Could you check a few things on this model? Use its own coordinates, in mm. A direction names the side the tool comes from. Round coordinates to 2 decimals unless told otherwise and drop trailing zeros. Loops run counter-clockwise (first coordinate to the right, second up) from the corner with the lowest first, then second, coordinate; pieces in that order, holes last. Notation, with made-up numbers: (-18, 38.5) -> (26, 38.5) arc R16 ccw to (26, 50.5) -> close; hole circle Ø5 at (26, 49.25). An arc over 180 degrees is marked (long way). Write each question's results on one line, items separated by ' | '. Start each with the question number.
1) Imagine slicing it at A-A, the plane y = 4.5. List the corners of the cut face in (x, z) for me.
2) Which directions (+Z, -Z, +X, -X, +Y, -Y) give clear straight access to the entire face, cutting with the end or side of a thin tool? Please do faces 4 (the flat face through (-2.642, 1, -7)), 5 (the flat face through (8, 9, -1.016)), 6 (the flat face through (6.706, 9.1, -0.5)).
3) Imagine slicing it at D-D, the plane z = -6. List the corners of the cut face in (x, y) for me.
4) For P1, Ø2, axis at x = 2, z = -3, coming from the +Y side, with a flat end and sliding along its axis, tell me the tip position at first contact or that it passes through.
5) If I drill on probe 1 along Z at (x, y) = (8.75, 11.5); probe 2 along Z at (x, y) = (4, 3.25); probe 3 along Y at (x, z) = (-1.5, -4), over which ranges is the centre line in solid material (lowest first)?
6) Imagine slicing it at C-C, the plane z = -0.25. List the corners of the cut face in (x, y) for me (3 decimals).
7) Imagine slicing it at B-B, the plane x = 1.5. List the corners of the cut face in (y, z) for me (3 decimals), plus the area to 3 significant figures.
8) We'd pull the mould along Z, two halves only. Please class faces 1 (the flat face through (-1, 9, -11.684)), 2 (the flat face through (3, 8, 5.08)), 3 (the flat face through (3, 0, -7)): pulls with the +Z half, pulls with the -Z half, needs draft (parallel to the pull), parting line crosses it, or undercut.
Autodesk Inventor part; units mm, degrees
ref_plane "YZ Plane" through (0, 0, 0) normal (1, 0, 0) x (0, 1, 0)
ref_plane "XZ Plane" through (0, 0, 0) normal (0, 1, 0) x (-1, 0, 0)
ref_plane "XY Plane" through (0, 0, 0) normal (0, 0, 1) x (1, 0, 0)
sketch "Sketch5" plane through (0, 0, 0) normal (0, 1, 0) x (-1, 0, 0)
  line L0 (0, 0) -> (-6.604, 0) construction
  line L1 (-6.604, 0) -> (-6.604, -12.7) construction
  line L2 (-6.604, -12.7) -> (0, -12.7) construction
  line L3 (0, -12.7) -> (0, 0) construction
  line L4 (2.6416, -15.24) -> (-9.2456, -15.24)
  line L5 (-9.2456, -15.24) -> (-9.2456, 2.54)
  line L6 (-9.2456, 2.54) -> (2.6416, 2.54)
  line L7 (2.6416, 2.54) -> (2.6416, -15.24)
  dimension "d22" = 6.604
  dimension "d23" = 12.7
  dimension "d24" = 2.6416
  dimension "d25" = 2.6416
  dimension "d26" = 2.54
  dimension "d27" = 2.54
extrude "Extrusion3" add sketch "Sketch5" along normal blind 2.54
sketch "Sketch6" plane through (0, 2.54, 0) normal (0, 1, 0) x (1, 0, 0)
  line L0 (-2.6416, -2.54) -> (9.2456, -2.54)
  line L1 (9.2456, -2.54) -> (9.2456, 0)
  line L2 (6.7056, 0) -> (-0.1016, 0)
  line L3 (-2.6416, -0.508) -> (-2.6416, -2.54)
  line L4 (-2.6416, 15.24) -> (-2.6416, -2.54)
  line L5 (9.2456, -2.54) -> (9.2456, 15.24)
  line L6 (-2.6416, -2.54) -> (9.2456, -2.54)
  line L7 (-0.1016, 12.7) -> (6.7056, 12.7)
  line L8 (9.2456, 12.954) -> (9.2456, 15.24)
  line L9 (9.2456, 15.24) -> (-2.6416, 15.24)
  line L10 (-2.6416, 15.24) -> (-2.6416, 12.7)
  line L11 (9.2456, 15.24) -> (-2.6416, 15.24)
  line L12 (9.2456, 12.954) -> (9.2456, 11.684)
  line L13 (6.7056, 11.684) -> (6.7056, 12.7)
  line L14 (6.7056, 11.684) -> (9.2456, 11.684)
  line L15 (-2.6416, 12.7) -> (-2.6416, 11.684)
  line L16 (-2.6416, 11.684) -> (-0.1016, 11.684)
  line L17 (-0.1016, 11.684) -> (-0.1016, 12.7)
  line L18 (9.2456, 0) -> (9.2456, 1.016)
  line L19 (9.2456, 1.016) -> (6.7056, 1.016)
  line L20 (6.7056, 1.016) -> (6.7056, 0)
  line L21 (-0.1016, 0) -> (-0.1016, 1.016)
  line L22 (-0.1016, 1.016) -> (-2.6416, 1.016)
  line L23 (-2.6416, 1.016) -> (-2.6416, -0.508)
  point P0 (0, 0)
  point P1 (7.9756, 11.684)
  point P2 (9.2456, 0.508)
  point P3 (-2.6416, 15.24)
  point P4 (-2.6416, 1.016)
  point P5 (9.2456, 0)
  dimension "d30" = 2.54
  dimension "d31" = 2.54
  dimension "d32" = 2.54
  dimension "d33" = 1.016
  dimension "d35" = 2.54
  dimension "d36" = 1.016
  dimension "d37" = 1.016
  dimension "d38" = 2.54
  dimension "d39" = 2.54
  dimension "d40" = 1.016
extrude "Extrusion4" add sketch "Sketch6" along normal blind 13.335 contours L3 L4 L22 L21 L2 L20 L19 L5 L1 L0 | L4 L9 L5 L14 L13 L7 L17 L16
sketch "Sketch8" plane through (9.2456, 0, -15.24) normal (0, 0, -1) x (-1, 0, 0)
  line L0 (0, 0) -> (0, 15.875)
  line L1 (11.8872, 0) -> (0, 0)
  line L2 (0, 15.875) -> (11.8872, 15.875)
  line L3 (11.8872, 15.875) -> (11.8872, 0)
  line L4 (11.8872, 0) -> (0, 0)
  line L5 (0, 0) -> (0, 15.875)
  point P0 (9.2456, 0)
extrude "Extrusion5" add sketch "Sketch8" along normal blind 2.54
sketch "Sketch9" plane through (-2.6416, 0, 2.54) normal (0, 0, 1) x (1, 0, 0)
  line L0 (2.54, 15.875) -> (0, 15.875)
  line L1 (11.8872, 0) -> (0, 0)
  line L2 (0, 15.875) -> (11.8872, 15.875)
  line L3 (11.8872, 15.875) -> (11.8872, 0)
  line L4 (11.8872, 0) -> (0, 0)
  line L5 (0, 0) -> (0, 15.875)
  point P0 (2.6416, 0)
  point P1 (0, 0)
extrude "Extrusion6" add sketch "Sketch9" along normal blind 2.54
properties part number "LatchSingleFit" material "PC/ABS Plastic"
Checked values:
1) outline: (-2.64, -17.78) -> (9.25, -17.78) -> (9.25, -11.68) -> (6.71, -11.68) -> (6.71, -12.7) -> (-0.1, -12.7) -> (-0.1, -11.68) -> (-2.64, -11.68) -> close; (-2.64, -1.02) -> (-0.1, -1.02) -> (-0.1, 0) -> (6.71, 0) -> (6.71, -1.02) -> (9.25, -1.02) -> (9.25, 5.08) -> (-2.64, 5.08) -> close
2) face 4: +Z, -Z, -X, +Y, -Y | face 5: +X, -X, +Y | face 6: +Y
3) outline: (-2.64, 0) -> (9.25, 0) -> (9.25, 2.54) -> (-2.64, 2.54) -> close
4) P1: y = 2.54
5) probe 1: -17.78 to -11.68, -1.02 to 5.08 | probe 2: -17.78 to -12.7, 0 to 5.08 | probe 3: 0 to 2.54
6) outline: (-2.642, 0) -> (9.246, 0) -> (9.246, 15.875) -> (6.706, 15.875) -> (6.706, 2.54) -> (-0.102, 2.54) -> (-0.102, 15.875) -> (-2.642, 15.875) -> close
7) outline: (0, -17.78) -> (15.875, -17.78) -> (15.875, -12.7) -> (2.54, -12.7) -> (2.54, 0) -> (15.875, 0) -> (15.875, 5.08) -> (0, 5.08) -> close | area: 194 mm^2
8) face 1: undercut | face 2: pulls with the +Z half | face 3: needs draft
